Autodesk Inventor part; units mm, degrees
ref_plane "YZ Plane" through (0, 0, 0) normal (1, 0, 0) x (0, 1, 0)
ref_plane "XZ Plane" through (0, 0, 0) normal (0, 1, 0) x (-1, 0, 0)
ref_plane "XY Plane" through (0, 0, 0) normal (0, 0, 1) x (1, 0, 0)
sketch "Sketch1" plane through (0, 0, 0) normal (0, 1, 0) x (-1, 0, 0)
  line L0 (-60, 92.5) -> (60, 92.5)
  line L1 (60, 92.5) -> (60, -92.5)
  line L2 (60, -92.5) -> (-60, -92.5)
  line L3 (-60, -92.5) -> (-60, 92.5)
  line L4 (-60, 92.5) -> (60, -92.5) construction
  line L5 (60, 92.5) -> (-60, -92.5) construction
  point P0 (0, 0)
  dimension "d0" = 120
  dimension "d1" = 185
extrude "Extrusion1" add sketch "Sketch1" along normal blind 5
sketch "Sketch2" plane through (0, 5, 0) normal (0, 1, 0) x (1, 0, 0)
  line L0 (55, -87.5) -> (-55, -87.5)
  line L1 (-55, -87.5) -> (-55, 87.5)
  line L2 (-55, 87.5) -> (55, 87.5)
  line L3 (55, 87.5) -> (55, -87.5)
  line L4 (55, -87.5) -> (-55, 87.5) construction
  line L5 (-55, -87.5) -> (55, 87.5) construction
  line L6 (50, -82.5) -> (-50, -82.5)
  line L7 (-50, -82.5) -> (-50, 82.5)
  line L8 (-50, 82.5) -> (50, 82.5)
  line L9 (50, 82.5) -> (50, -82.5)
  line L10 (50, -82.5) -> (-50, 82.5) construction
  line L11 (-50, -82.5) -> (50, 82.5) construction
  point P0 (0, 0)
  dimension "d4" = 110
  dimension "d5" = 175
  dimension "d6" = 100
  dimension "d7" = 165
extrude "Extrusion2" add sketch "Sketch2" along normal blind 5
sketch "Sketch4" plane through (0, 5, 0) normal (0, 1, 0) x (1, 0, 0)
  circle A0 centre (57.5, -90) radius 1.625
  circle A1 centre (57.5, 90) radius 1.625
  circle A2 centre (-57.5, 90) radius 1.625
  circle A3 centre (-57.5, -90) radius 1.625
  point P0 (0, 0)
  dimension "d11" = 3.25
  dimension "d12" = 3.25
  dimension "d13" = 3.25
  dimension "d16" = 3.25
extrude "Extrusion3" cut sketch "Sketch4" against normal blind 5
sketch "Sketch5" plane through (0, 5, 0) normal (0, 1, 0) x (1, 0, 0)
  circle A0 centre (57.5, 90) radius 1.625
  circle A1 centre (57.5, 90) radius 1.625
  circle A2 centre (57.5, -90) radius 1.625
  circle A3 centre (57.5, -90) radius 1.625
  circle A4 centre (-57.5, -90) radius 1.625
  circle A5 centre (-57.5, -90) radius 1.625
  circle A6 centre (-57.5, 90) radius 1.625
  circle A7 centre (-57.5, 90) radius 1.625
  point P0 (0, 0)
extrude "Extrusion4" add sketch "Sketch5" against normal blind 2
sketch "Sketch6" plane through (0, 5, 0) normal (0, 1, 0) x (1, 0, 0)
  circle A0 centre (57.5, 90) radius 1.625
  circle A1 centre (57.5, 90) radius 0.75
  circle A2 centre (57.5, -90) radius 1.625
  circle A3 centre (57.5, -90) radius 0.75
  circle A4 centre (-57.5, -90) radius 1.625
  circle A5 centre (-57.5, -90) radius 0.75
  circle A6 centre (-57.5, 90) radius 1.625
  circle A7 centre (-57.5, 90) radius 0.75
  point P0 (0, 0)
  dimension "d19" = 1.5
  dimension "d20" = 1.5
  dimension "d21" = 1.5
  dimension "d22" = 1.5
extrude "Extrusion5" cut sketch "Sketch6" against normal blind 2 contours A1 | A3 | A5 | A7
properties part number "Enclose Bottom" material "PC/ABS Plastic"
Part model, mm, in its own coordinate system. A direction names the side the tool comes from. Round coordinates to 2 decimals unless told otherwise and drop trailing zeros. Order: outer loops, then holes, each group sorted by start corner. A loop starts at its lowest first (then second) coordinate and runs counter-clockwise, first axis right, second up. Notation, with made-up numbers: M -33,27 L -2,27 A23 cw -2,43 Z; hole C -31,82.25 d5. An arc over 180 degrees is marked long. Put each result on its own line as item: value. Start each with the question number.
1. Two-plate mould, pull along Z, no slides. Class faces 4 (the face through (-55, 7, 1)), 5 (the face through (-1, 7, -82.5)), 6 (the face through (-50, 7, 1)), 7 (the face through (-1, 2, -92.5)): +Z half, -Z half, draft (parallel to the pull), parting line (faces both ways), or undercut.
2. Tool access for faces 1 (the face through (-1, 7, -87.5)), 2 (the face through (50, 7, -1)), 3 (the face through (1, 7, 87.5)): list every direction of +Z, -Z, +X, -X, +Y, -Y with a clear straight run to the whole face (end or side of a thin tool).
3. Slice it at C-C on z = 43. List the corners of the cut face in (x, y), then the cut area to 3 significant figures.
4. Slice it at B-B on y = 7.5. List the corners of the cut face in (x, z), then the cut area to 3 significant figures.
5. Drop flat-ended pins along their axis: pin 1 (2.5 mm diameter, centred on x = -9, y = 8, fed in from +Z); pin 2 (5.5 mm diameter, centred on y = 8.5, z = 20.5, fed in from +X); pin 3 (3.5 mm diameter, centred on x = 57, z = 90, fed in from -Y); pin 4 (2 mm diameter, centred on x = 13, y = 8.5, fed in from -Z). Give the stop position or say it passes through.
6. Drill centre lines: probe 1 along X at (y, z) = (4.45, 90); probe 2 along Z at (x, y) = (-57.5, 2.05) (3 decimals); probe 3 along X at (y, z) = (1.3, 90) (3 decimals). Where is each one in solid material? Low to high. Write a range as [from, to].
7. Slice it at A-A on x = -41.5. List the corners of the cut face in (y, z), then the cut area to 3 significant figures.
Findings:
1. face 4: draft
1. face 5: undercut
1. face 6: undercut
1. face 7: -Z half
2. face 1: -Z, +X, -X, +Y
2. face 2: +Y
2. face 3: +Z, +X, -X, +Y
3. outline: M -60,0 L 60,0 L 60,5 L 55,5 L 55,10 L 50,10 L 50,5 L -50,5 L -50,10 L -55,10 L -55,5 L -60,5 Z
3. area: 650 mm2
4. outline: M -55,-87.5 L 55,-87.5 L 55,87.5 L -55,87.5 Z; hole M -50,-82.5 L 50,-82.5 L 50,82.5 L -50,82.5 Z
4. area: 2,750 mm2
5. pin 1: z = 87.5
5. pin 2: x = 55
5. pin 3: y = 0
5. pin 4: z = -87.5
6. probe 1: [-60, -58.25], [-56.75, 56.75], [58.25, 60]
6. probe 2: [-92.5, -91.625], [-88.375, 88.375], [91.625, 92.5]
6. probe 3: [-60, -59.125], [-55.875, 55.875], [59.125, 60]
7. outline: M 0,-92.5 L 5,-92.5 L 5,-87.5 L 10,-87.5 L 10,-82.5 L 5,-82.5 L 5,82.5 L 10,82.5 L 10,87.5 L 5,87.5 L 5,92.5 L 0,92.5 Z
7. area: 975 mm2
